The model under review builds one solid part; all positions refer to its coordinate system, in mm. A direction names the side the tool comes from. Coordinates: 2 decimals unless noted, no trailing zeros. Order: outer loops, then holes, each group sorted by start corner. A loop starts at its lowest first (then second) coordinate and runs counter-clockwise, first axis right, second up. Notation, with made-up numbers: M 41.25,-29.5 L 93.25,-29.5 A13 cw 93.25,-11.5 Z; hole C -24,81.5 d8. An arc over 180 degrees is marked long. One line per item, written item: value.
```python
from build123d import *

# Parameters (mm, degrees)
F2_W          = 193.8
F2_H          = 44.1753827035
F3_DEPTH      = 43.601
F3_DEPTH_BACK = 43.601
F5_D          = 20
F6_SIZE       = 3


with BuildPart() as f1:
    # F0 (on Front) → F1 (revolve)
    with BuildSketch(Plane.XZ):
        Polygon((-158.8, 18.75), (-158.8, 0), (232, 0), (232, 28), (0, 28), (0, 43.6), (-24, 43.6), (-24, 28), (-113.8, 28), (-113.8, 18.75), align=None)
    revolve(axis=Axis((36.6, 0, 0), (-1, 0, 0)))

    # F2 (on Front) → F3 (cut, two sides)
    with BuildSketch(Plane.XZ) as f3_sk:
        with Locations((120, 18.9876913518)):
            Rectangle(F2_W, F2_H)
    extrude(amount=-F3_DEPTH, mode=Mode.SUBTRACT)
    extrude(f3_sk.sketch, amount=F3_DEPTH_BACK, mode=Mode.SUBTRACT)

    # F5 (through all)
    with Locations(Plane.XY.offset(-3.1)):
        with Locations((70, 0), (170, 0)):
            Hole(F5_D / 2)

    # F6
    f6_edges = [f1.edges().sort_by_distance(p)[0] for p in [
        (-158.8, 0, -18.75),
    ]]
    chamfer(f6_edges, length=F6_SIZE)


solid = f1.part
```
(1) We need section A-A, the plane x = 172. State the section outline as (y, z) points, plus the area to 3 significant figures.
Geometry results:
outline: M -27.83,-3.1 A28 ccw -9.8,-26.23 L -9.8,-3.1 Z; M 9.8,-26.23 A28 ccw 27.83,-3.1 L 9.8,-3.1 Z
area: 582 mm2
(2) Tool access review of faces 5 (the flat face through (23.1, 0, 9)), 6 (the cylindrical face through (-69.529, -10.724, 25.865)), 7 (the cylindrical face through (114.376, 1.231, -27.973)), 8 (the flat face through (-158.8, 0, 0)): name each direction out of +Z, -Z, +X, -X, +Y, -Y from which nothing blocks a thin tool from reaching the whole face with its end or side.
Geometry results:
face 5: +Z, +Y, -Y
face 6: -X
face 7: +X
face 8: +Z, -Z, -X, +Y, -Y
(3) Insertion check: pin 1 Ø8 at (x, z) = (81.5, -18) entering from +Y; pin 2 Ø23 at (x, y) = (170, 0) entering from -Z; pin 3 Ø12 at (x, y) = (23, -6) entering from +Z. Each pin has a flat end and moves straight along its axis. Give the tip position at first contact, or say it passes through.
Geometry results:
pin 1: stops at y = 24.25
pin 2: stops at z = -28
pin 3: stops at z = 28
(4) We need section B-B, the plane x = -43.5. State the section outline as (y, z) points, plus the area to 3 significant figures.
Geometry results:
outline: C 0,0 d56
area: 2,460 mm2
(5) For L1, parallel to X at y = 0, z = -15; L2, parallel to X at y = 22.5, z = 13.5; L3, parallel to X at y = 31, z = -8, list the stretches that pass through material, from the lowest coordinate up.
Geometry results:
L1: x = -158.8 to 60, 80 to 160, 180 to 232
L2: x = -113.8 to 23.1, 216.9 to 232
L3: x = -24 to 0
(6) Mouldability with a two-part tool opening along X and no side actions: class faces 1 (the flat face through (-24, -28.5, -0.6)), 2 (the flat face through (119, 0, -3.1)), 3 (the cylindrical face through (-12.168, 13.096, 41.587)), 4 (the flat face through (216.9, 0, 9)) as +X half, -X half, draft (parallel to the pull), parting line (faces both ways), or undercut.
Geometry results:
face 1: -X half
face 2: undercut
face 3: draft
face 4: undercut
(7) We need section C-C, the plane y = 5.5. Count the separate pieces of the cut face and the enclosed holes in it, plus the area to 3 significant figures.
Geometry results:
separate pieces: 3
enclosed holes: 0
area: 14,600 mm2
(8) We need section D-D, the plane z = 38. State the section outline as (x, y) points, plus the area to 3 significant figures.
Geometry results:
outline: M -24,-21.38 L 0,-21.38 L 0,21.38 L -24,21.38 Z
area: 1,030 mm2
